Verification items for the finished model (mm, model axes). Face numbers are marked on the shaded views. A direction names the side the tool comes from. Coordinates: 2 decimals unless noted, no trailing zeros. Write each loop counter-clockwise with the first axis right and the second up, starting at its lowest first coordinate (ties: lowest second). Pieces come first, ordered by that corner, then holes. Notation, with made-up numbers: M -7,79.25 L 11,79.25 A11 ccw 11,86.25 Z; hole C -16.5,40.5 d8. An arc over 180 degrees is marked long. Answer in a Markdown table with one row per item.
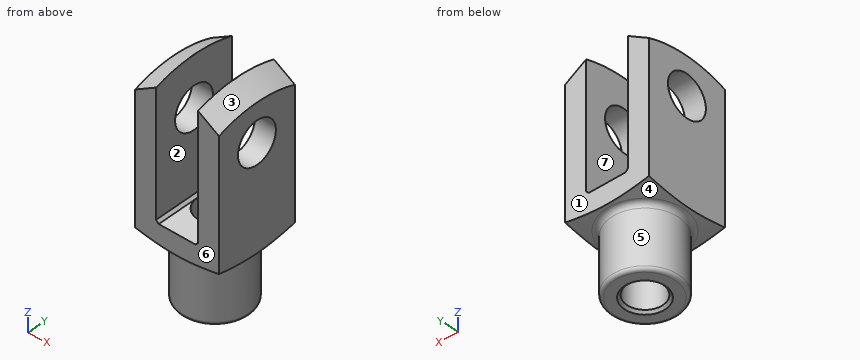
from build123d import *

# Parameters (mm, degrees)
CUT_EXTRUDE1_DEPTH           = 33
CUT_EXTRUDE1_DEPTH_BACK      = 33
CUT_EXTRUDE2_DEPTH           = 33
CUT_EXTRUDE2_DEPTH_BACK      = 33
CUT_EXTRUDE3_DEPTH           = 33
CUT_EXTRUDE3_DEPTH_BACK      = 33
SKETCH5_W                    = 39.5
SKETCH5_H                    = 8
CUT_REVOLVE3_ANGLE           = 90
CUT_REVOLVE3_OTHER_WAY_ANGLE = 90


with BuildPart() as part:
    # Sketch1 → Revolve1 (revolve)
    with BuildSketch(Plane(origin=(0, 0, 0), x_dir=(0, 0, -1), z_dir=(1, 0, 0))):
        with BuildLine():
            Line((-19, 0), (-19, 32))
            Line((-19, 32), (35.444863729, 32))
            Line((35.444863729, 32), (40, 15))
            ThreePointArc((40, 15), (40.585786438, 13.585786438), (42, 13))
            Line((42, 13), (62.7, 13))
            ThreePointArc((62.7, 13), (63.619238816, 12.619238816), (64, 11.7))
            Line((64, 11.7), (64, 0))
            Line((64, 0), (-19, 0))
        make_face()
    revolve(axis=Axis((0, 0, -64), (0, 0, 1)))

    # Sketch2 → Cut-Extrude1 (cut, two sides)
    with BuildSketch(Plane(origin=(0, 0, 0), x_dir=(1, 0, 0), z_dir=(0, 1, 0))) as cut_extrude1_sk:
        Polygon((-8, 31), (-8, -20), (8, -20), (8, 31), (7, 32), (-7, 32), align=None)
    extrude(amount=CUT_EXTRUDE1_DEPTH, mode=Mode.SUBTRACT)
    extrude(cut_extrude1_sk.sketch, amount=-CUT_EXTRUDE1_DEPTH_BACK, mode=Mode.SUBTRACT)

    # Sketch3 → Cut-Extrude2 (cut, two sides)
    with BuildSketch(Plane(origin=(0, 0, 0), x_dir=(0, 0, -1), z_dir=(1, 0, 0))) as cut_extrude2_sk:
        Polygon((-52, -48), (64, -48), (64, -16), (-20, -16), (-20, 16), (64, 16), (64, 48), (-52, 48), align=None)
    extrude(amount=CUT_EXTRUDE2_DEPTH, mode=Mode.SUBTRACT)
    extrude(cut_extrude2_sk.sketch, amount=-CUT_EXTRUDE2_DEPTH_BACK, mode=Mode.SUBTRACT)

    # Sketch4 → Cut-Extrude3 (cut, two sides)
    with BuildSketch(Plane(origin=(0, 0, 0), x_dir=(1, 0, 0), z_dir=(0, 1, 0))) as cut_extrude3_sk:
        Polygon((-48, -52), (48, -52), (48, 64), (16, 64), (16, -20), (-16, -20), (-16, 64), (-48, 64), align=None)
    extrude(amount=CUT_EXTRUDE3_DEPTH, mode=Mode.SUBTRACT)
    extrude(cut_extrude3_sk.sketch, amount=-CUT_EXTRUDE3_DEPTH_BACK, mode=Mode.SUBTRACT)

    # Sketch5 → Cut-Revolve1 (revolve, cut)
    with BuildSketch(Plane.XY):
        with Locations((0, 4)):
            Rectangle(SKETCH5_W, SKETCH5_H)
    revolve(axis=Axis((19.75, 0, 0), (-1, 0, 0)), mode=Mode.SUBTRACT)

    # Sketch6 → Cut-Revolve2 (revolve, cut)
    with BuildSketch(Plane(origin=(0, 0, 0), x_dir=(0, 0, -1), z_dir=(1, 0, 0))):
        Polygon((30.9, 0), (30.9, 6.9175), (63.0175, 6.9175), (64.1, 8), (64.1, 0), align=None)
    revolve(axis=Axis((0, 0, -64.1), (0, 0, 1)), mode=Mode.SUBTRACT)

    # Sketch7 → Cut-Revolve3 (revolve, cut)
    with BuildSketch(Plane(origin=(0, 0, 0), x_dir=(1, 0, 0), z_dir=(0, 1, 0))):
        Polygon((-19, -49.64182924), (0, -60.611484355), (19, -49.64182924), (19, -12.691412012), (0, -23.661067127), (-19, -12.691412012), align=None)
    revolve(axis=Axis((-19, 0, -32), (1, 0, 0)), revolution_arc=CUT_REVOLVE3_ANGLE, mode=Mode.SUBTRACT)

    # Sketch7 → Cut-Revolve3 other way (revolve, cut)
    with BuildSketch(Plane(origin=(0, 0, 0), x_dir=(1, 0, 0), z_dir=(0, 1, 0))):
        Polygon((-19, -49.64182924), (0, -60.611484355), (19, -49.64182924), (19, -12.691412012), (0, -23.661067127), (-19, -12.691412012), align=None)
    revolve(axis=Axis((-19, 0, -32), (-1, 0, 0)), revolution_arc=CUT_REVOLVE3_OTHER_WAY_ANGLE, mode=Mode.SUBTRACT)


solid = part.part
1) Sectioned sample at D-D (z = 0). Record the cut outline in (x, y).
Response values:
| item | result |
|---|---|
| outline | M -16,-16 L -8,-16 L -8,-8 L -16,-8 Z; M -16,8 L -8,8 L -8,16 L -16,16 Z; M 8,-16 L 16,-16 L 16,-8 L 8,-8 Z; M 8,8 L 16,8 L 16,16 L 8,16 Z |
2) Release check for a two-part mould opening along X. For the marked faces 1, 2, 3 and 4 record: +X half, -X half, draft (parallel to the pull), parting line (faces both ways), or undercut.
Response values:
| item | result |
|---|---|
| face 1 | draft |
| face 2 | undercut |
| face 3 | +X half |
| face 4 | parting line |
3) Depth check by flat-ended pin: pin 1 (11 mm diameter, centred on x = -2, y = 3.5, fed in from +Z); pin 2 (14.5 mm diameter, centred on y = 0, z = 0, fed in from -X); pin 3 (5 mm diameter, centred on y = 5, z = -53, fed in from -X); pin 4 (8 mm diameter, centred on y = 7.5, z = -54.5, fed in from +X). Enter the tip coordinate at first touch or a pass-through.
Response values:
| item | result |
|---|---|
| pin 1 | stops at z = -31.5 |
| pin 2 | passes through |
| pin 3 | stops at x = -12.76 |
| pin 4 | stops at x = 12.52 |
4) Tool access check on the marked faces 5, 6 and 7. Record the directions out of +Z, -Z, +X, -X, +Y, -Y that give a thin tool (end or side, any length) a straight path to the whole face; none if there is none.
Response values:
| item | result |
|---|---|
| face 5 | -Z |
| face 6 | +Z, -Z, +X, -X, -Y |
| face 7 | +Z, +Y, -Y |
5) Sectioned sample at C-C (y = 0). Give the number of separate pieces and of enclosed holes in the cut face, then the cut area to 3 significant figures.
Response values:
| item | result |
|---|---|
| separate pieces | 4 |
| enclosed holes | 0 |
| area | 962 mm² |
6) Sectioned sample at B-B (x = 0). Record the cut outline in (y, z), then the cut area to 3 significant figures.
Response values:
| item | result |
|---|---|
| outline | M -16,-39.73 L -15,-40 A2 cw -13,-42 L -13,-62.7 A1.3 ccw -11.7,-64 L -7.9,-64 L -6.92,-63.02 L -6.92,-32 L -16,-32 Z; M 6.92,-63.02 L 7.9,-64 L 11.7,-64 A1.3 ccw 13,-62.7 L 13,-42 A2 cw 15,-40 L 16,-39.73 L 16,-32 L 6.92,-32 Z |
| area | 437 mm² |
7) Sectioned sample at A-A (z = -29.5). Record the cut outline in (x, y).
Response values:
| item | result |
|---|---|
| outline | M -16,-16 L -8,-16 L -8,16 L -16,16 Z; M 8,-16 L 16,-16 L 16,16 L 8,16 Z |
8) Thickness scan on L1, parallel to X at y = 0, z = -51.5; L2, parallel to X at y = 4, z = -10.5; L3, parallel to Y at x = 12, z = -0.5. Record the ranges inside material, lowest first. Write a range as [from, to].
Response values:
| item | result |
|---|---|
| L1 | x = [-13, -6.92], [6.92, 13] |
| L2 | x = [-16, -8], [8, 16] |
| L3 | y = [-16, -7.98], [7.98, 16] |
